Autodesk Inventor part; units mm, degrees
ref_plane "YZ Plane" through (0, 0, 0) normal (1, 0, 0) x (0, 1, 0)
ref_plane "XZ Plane" through (0, 0, 0) normal (0, 1, 0) x (-1, 0, 0)
ref_plane "XY Plane" through (0, 0, 0) normal (0, 0, 1) x (1, 0, 0)
sketch "スケッチ1" plane through (0, 0, 0) normal (0, 0, 1) x (1, 0, 0)
  circle A0 centre (0, 0) radius 19.25
  dimension "d0" = 38.5
extrude "押し出し1" add sketch "スケッチ1" along normal blind 57
sketch "スケッチ2" plane through (0, 0, 57) normal (0, 0, 1) x (1, 0, 0)
  circle A0 centre (0, 0) radius 16
  dimension "d3" = 32
extrude "押し出し2" add sketch "スケッチ2" along normal blind 34.9
sketch "スケッチ3" plane through (0, 0, 91.9) normal (0, 0, 1) x (1, 0, 0)
  circle A0 centre (0, 0) radius 3
  dimension "d6" = 6
extrude "押し出し3" add sketch "スケッチ3" along normal blind 19.3
sketch "スケッチ4" plane through (0, 0, 91.9) normal (0, 0, 1) x (1, 0, 0)
  circle A0 centre (0, 0) radius 3
  circle A1 centre (0, 0) radius 10
  dimension "d9" = 20
extrude "押し出し4" add sketch "スケッチ4" along normal blind 3
sketch "スケッチ5" plane through (0, 0, 91.9) normal (0, 0, 1) x (1, 0, 0)
  circle A0 centre (0, 0) radius 3
  circle A1 centre (0, 0) radius 13
  point P0 (0, 13)
  point P1 (-13, 0)
  point P2 (0, -13)
  point P3 (13, 0)
  dimension "d12" = 26
  dimension "d15" = 360
hole "穴1" at (0, 13, 91.9) at (-13, 0, 91.9) at (0, -13, 91.9) at (13, 0, 91.9) direction (0, 0, -1) diameter 3 depth 4 tip angle 118
properties part number "rs555vc5524"
The model under review builds one solid part; all positions refer to its coordinate system, in mm. A direction names the side the tool comes from. Coordinates: 2 decimals unless noted, no trailing zeros. Write each loop counter-clockwise with the first axis right and the second up, starting at its lowest first coordinate (ties: lowest second). Pieces come first, ordered by that corner, then holes. Notation, with made-up numbers: (51, 75.5) -> (96, 75.5) arc R24 ccw to (96, 90.5) -> close; hole circle Ø6 at (3, 9). An arc over 180 degrees is marked (long way). One line per item, written item: value. Start each with the question number.
Q1. The part is to be moulded in two halves that separate along Y. For faces 1 (the face through (-0.2, -10.4, 91.9)), 2 (the face through (-0.07, -11.5, 89.87)), 3 (the face through (-3.47, 15.62, 74.21)), say which applies: +Y half, -Y half, draft (parallel to the pull), parting line (faces both ways), or undercut.
Q2. Clearance check with flat-ended pins moving along their axes: P1, Ø6, axis at x = 5, y = 1.5, coming from the +Z side; P2, Ø5, axis at x = 2.5, z = 35.5, coming from the -Y side; P3, Ø12, axis at x = -7, z = 58, coming from the +Y side; P4, Ø3, axis at y = -10.5, z = 84.5, coming from the +X side. State where each tip first meets the part, or that it passes through.
Q3. To check wall thickness, follow probe 1 along Y at (x, z) = (0, 88); probe 2 along Z at (x, y) = (17.5, -6.5); probe 3 along Z at (x, y) = (-10, 4.5). State the ranges of each line that lie inside material, in increasing order.
Q4. Add section D-D, the plane x = 8. Give the boundary of the cut face in (y, z), then the cut area to 3 significant figures.
Q5. For faces 4 (the face through (0, 0, 111.2)), 5 (the face through (-3, 0, 103)), list the 3-axis set-ups (+Z, -Z, +X, -X, +Y, -Y) from which the entire face can be reached by the end or side of a thin tool; tool diameter is ignored.
Q6. Add section A-A, the plane z = 48.5. Give the boundary of the cut face in (x, y).
Q7. Add section B-B, the plane x = -7.5. Give the boundary of the cut face in (y, z), then the cut area to 3 significant figures.
Q8. Add section C-C, the plane z = 75. Give the boundary of the cut face in (x, y), then the cut area to 3 significant figures.
Response:
1. face 1: draft
1. face 2: undercut
1. face 3: parting line
2. P1: z = 111.2
2. P2: y = -19.25
2. P3: y = 19.22
2. P4: x = 13.23
3. probe 1: -16 to -14.5, -11.5 to 11.5, 14.5 to 16
3. probe 2: 0 to 57
3. probe 3: 0 to 91.9
4. outline: (-17.51, 0) -> (17.51, 0) -> (17.51, 57) -> (13.86, 57) -> (13.86, 91.9) -> (6, 91.9) -> (6, 94.9) -> (-6, 94.9) -> (-6, 91.9) -> (-13.86, 91.9) -> (-13.86, 57) -> (-17.51, 57) -> close
4. area: 3,000 mm²
5. face 4: +Z, +X, -X, +Y, -Y
5. face 5: +Z
6. outline: circle Ø38.5 at (0, 0)
7. outline: (-17.73, 0) -> (17.73, 0) -> (17.73, 57) -> (14.13, 57) -> (14.13, 91.9) -> (6.61, 91.9) -> (6.61, 94.9) -> (-6.61, 94.9) -> (-6.61, 91.9) -> (-14.13, 91.9) -> (-14.13, 57) -> (-17.73, 57) -> close
7. area: 3,050 mm²
8. outline: circle Ø32 at (0, 0)
8. area: 804 mm²
